Answer from the drawing. Dimensions are ordinates in mm from the lowest x, y and z of the part. Round coordinates to 2 decimals unless told otherwise and drop trailing zeros. Loops run counter-clockwise (first coordinate to the right, second up) from the corner with the lowest first, then second, coordinate; pieces in that order, holes last.
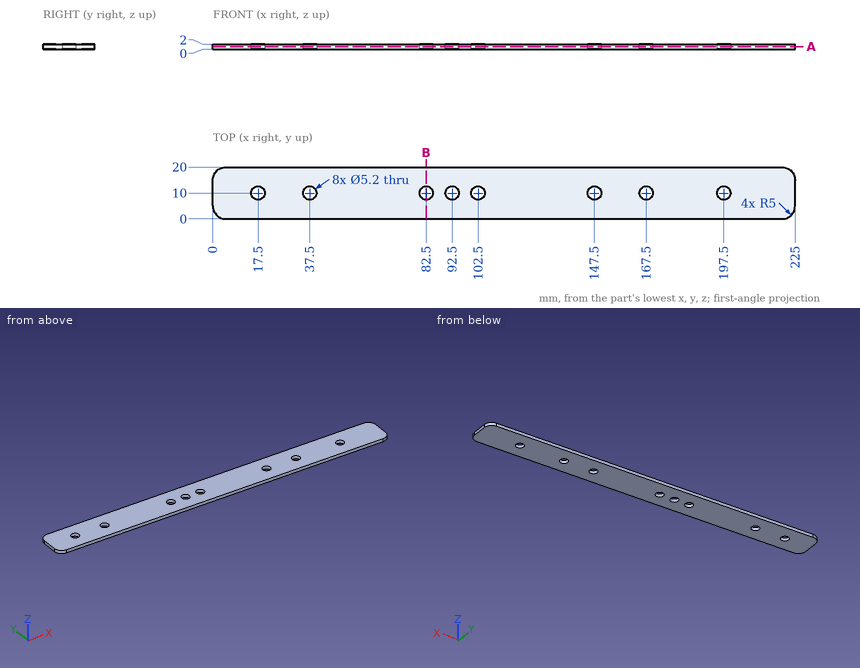
Item 1: Straight lines are drawn through the part: line 1 (Y direction, x = 17.5, z = 1.15); line 2 (Y direction, x = 16, z = 0.55); line 3 (X direction, y = 18.75, z = 0.35). For each, find the intervals that lie inside material, in ascending order.
Item 2: Section A-A, the plane z = 1 is taken. State how many separate pieces and enclosed holes the cut face has, plus the area to 3 significant figures.
Item 3: Section B-B, the plane x = 82.5 is taken. Give the vertices of the cut face in (y, z), plus the area to 3 significant figures.
Answer below:
1. line 1: y = 0 to 7.4, 12.6 to 20
1. line 2: y = 0 to 7.88, 12.12 to 20
1. line 3: x = 1.69 to 223.31
2. separate pieces: 1
2. enclosed holes: 8
2. area: 4,310 mm2
3. outline: (0, 0) - (7.4, 0) - (7.4, 2) - (0, 2) - close; (12.6, 0) - (20, 0) - (20, 2) - (12.6, 2) - close
3. area: 29.6 mm2
